Input: part model. Units: mm. Frame: model coordinates. Face numbers are marked on the shaded views. A direction names the side the tool comes from. Round coordinates to 2 decimals unless told otherwise and drop trailing zeros. Write each loop counter-clockwise with the first axis right and the second up, starting at its lowest first coordinate (ties: lowest second). Pieces come first, ordered by that corner, then holes. Notation, with made-up numbers: M 28,3 L 66,3 A8 ccw 66,16 Z; hole C 2,39 d4. An arc over 180 degrees is marked long. Use one line per item in the form item = value. Start each with the question number.
```python
from build123d import *

# Parameters (mm, degrees)
SKETCH1_R               = 20.7264
BOSS_EXTRUDE1_DEPTH     = 9.525
SKETCH2_R               = 5.5626
CUT_EXTRUDE1_DEPTH      = 7.9375
CIRPATTERN1_COUNT       = 4
SKETCH3_R               = 4.7625
BOSS_EXTRUDE2_DEPTH     = 77.47
CUT_EXTRUDE2_DEPTH      = 83.8297544
CUT_EXTRUDE2_DEPTH_BACK = 83.8297544
SKETCH5_R               = 1.5
SKETCH6_R               = 3.175
CUT_EXTRUDE3_DEPTH      = 85.316401939
CIRPATTERN2_COUNT       = 4
CHAMFER1_SIZE           = 0.635


with BuildPart() as part:
    # Sketch1 → Boss-Extrude1 (new body)
    with BuildSketch(Plane(origin=(0, 0, 0), x_dir=(1, 0, 0), z_dir=(0, 1, 0))):
        with Locations(Location((0, 0, 0), (0, 0, 90))):
            Circle(SKETCH1_R)
    extrude(amount=BOSS_EXTRUDE1_DEPTH)

    # Sketch2 → Cut-Extrude1 (cut)
    with BuildSketch(Plane(origin=(0, 9.525, 0), x_dir=(1, 0, 0), z_dir=(0, 1, 0))):
        with Locations(Location((0, 12.7, 0), (0, 0, 270))):
            Circle(SKETCH2_R)
    cut_extrude1 = extrude(amount=-CUT_EXTRUDE1_DEPTH, mode=Mode.SUBTRACT)

    # CirPattern1: Cut-Extrude1 ×4 about axis
    cirpattern1_axis = Axis((0, 0, 0), (0, 1, 0))
    for i in range(1, CIRPATTERN1_COUNT):
        add(cut_extrude1.rotate(cirpattern1_axis, i * 360 / CIRPATTERN1_COUNT), mode=Mode.SUBTRACT)

    # Sketch3 → Boss-Extrude2 (add)
    with BuildSketch(Plane.XZ):
        with Locations(Location((0, 0, 0), (0, 0, 270))):
            Circle(SKETCH3_R)
    extrude(amount=BOSS_EXTRUDE2_DEPTH)

    # Sketch4 → Revolve1 (revolve)
    with BuildSketch(Plane.XY, mode=Mode.PRIVATE) as revolve1_sk:
        Polygon((-20.7264, 0), (-4.7625, -6.35), (-4.7625, 0), align=None)
    revolve(revolve1_sk.sketch.rotate(Axis((0, 0, 0), (0, -1, 0)), 270), axis=Axis((0, 0, 0), (0, -1, 0)))

    # Sketch5 → Cut-Extrude2 (cut, two sides: drawn at the far end of the back side and taken through both)
    with BuildSketch(Plane.XY.offset(-CUT_EXTRUDE2_DEPTH_BACK)):
        with Locations((0, -71.12)):
            Circle(SKETCH5_R)
        with Locations((0, -61.595)):
            Circle(SKETCH5_R)
    extrude(amount=CUT_EXTRUDE2_DEPTH + CUT_EXTRUDE2_DEPTH_BACK, mode=Mode.SUBTRACT)

    # Sketch6 → Cut-Extrude3 (cut, through all)
    with BuildSketch(Plane(origin=(0, 1.5875, 0), x_dir=(1, 0, 0), z_dir=(0, 1, 0))):
        with Locations(Location((-12.7, 0, 0), (0, 0, 270))):
            Circle(SKETCH6_R)
    cut_extrude3 = extrude(amount=-CUT_EXTRUDE3_DEPTH, mode=Mode.SUBTRACT)

    # CirPattern2: Cut-Extrude3 ×4 about axis
    cirpattern2_axis = Axis((0, 0, 0), (0, 1, 0))
    for i in range(1, CIRPATTERN2_COUNT):
        add(cut_extrude3.rotate(cirpattern2_axis, i * 360 / CIRPATTERN2_COUNT), mode=Mode.SUBTRACT)

    # Chamfer1
    chamfer1_edges = [part.edges().sort_by_distance(p)[0] for p in [
        (0, -77.47, 4.7625),
    ]]
    chamfer(chamfer1_edges, length=CHAMFER1_SIZE)


solid = part.part
```
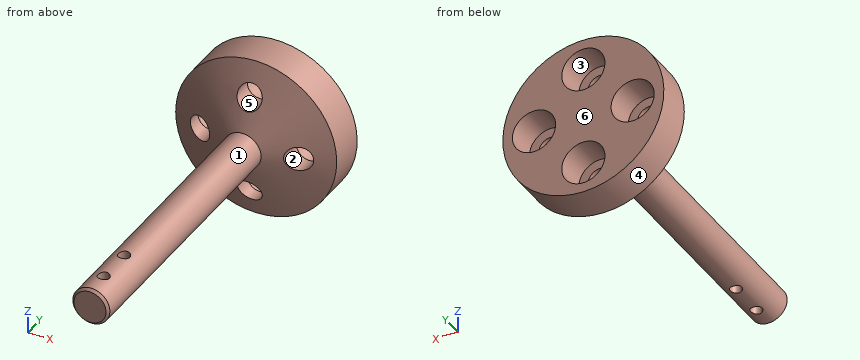
Item 1: First-contact query: pin 1 (5 mm diameter, centred on x = -4, y = -39, fed in from -Z); pin 2 (4 mm diameter, centred on x = 12.7, z = 0, fed in from +Y); pin 3 (3.5 mm diameter, centred on x = -14.5, z = -3, fed in from +Y); pin 4 (1 mm diameter, centred on x = -9, z = -5.5, fed in from -Y). Flat tips, straight axial feed; report the tip coordinate or a pass-through.
Item 2: Cut plane C-C (y = -71.12). Output: boundary loops of the cut face in (x, z) (1 decimal), plus the area to 3 significant figures.
Item 3: Ray query, line 1 (Y direction, x = 0, z = 0) (3 decimals); line 2 (X direction, y = 5.25, z = -12.7); line 3 (X direction, y = -12, z = 0). Return the intervals inside material, ascending. Write a range as from..to.
Item 4: Reachability of the marked faces 1, 2 and 3 from +Z, -Z, +X, -X, +Y, -Y: full face, straight path, thin tool, end or side. Return the list, or none.
Item 5: Cut plane A-A (y = 2.5). Output: boundary loops of the cut face in (x, z).
Item 6: Draft query along X for the marked faces 4, 5 and 6. Return one class per face: +X half, -X half, draft (parallel to the pull), parting line (faces both ways), or undercut.
Item 7: Cut plane B-B (y = -49.5). Output: boundary loops of the cut face in (x, z) (1 decimal), plus the area to 3 significant figures.
Final values:
q1.pin_1 = -4.52
q1.pin_2 = through
q1.pin_3 = 1.59
q1.pin_4 = -4.25
q2.outline = M -1.5,-4.5 L -1.5,4.5 A4.8 ccw Z; M 1.5,-4.5 A4.8 ccw 1.5,4.5 Z
q2.area = 43.2 mm^2
q3.line_1 = -77.47..-72.62, -69.62..-63.095, -60.095..9.525
q3.line_2 = -16.38..-5.56, 5.56..16.38
q3.line_3 = -4.76..4.76
q4.face_1 = -Y
q4.face_2 = +Y, -Y
q4.face_3 = +Y
q5.outline = C 0,0 d41.45; hole C -12.7,0 d11.13; hole C 0,-12.7 d11.13; hole C 0,12.7 d11.13; hole C 12.7,0 d11.13
q6.face_4 = parting line
q6.face_5 = undercut
q6.face_6 = draft
q7.outline = C 0,0 d9.5
q7.area = 71.3 mm^2
